Input: dimensioned drawing with shaded views. Units: mm. Origin: part minimum x, y, z. A direction names the side the tool comes from. Give positions to 0.01 mm unless a question says otherwise; leave off trailing zeros. Write each loop counter-clockwise with the first axis right and the second up, starting at its lowest first coordinate (ties: lowest second). Pieces come first, ordered by that corner, then holes. Notation, with made-up numbers: M 76.25,67.5 L 116.25,67.5 A22 cw 116.25,81.5 Z; hole C 8.25,8 d4. An arc over 180 degrees is marked long. Answer as a JSON object with one key per item and string values.
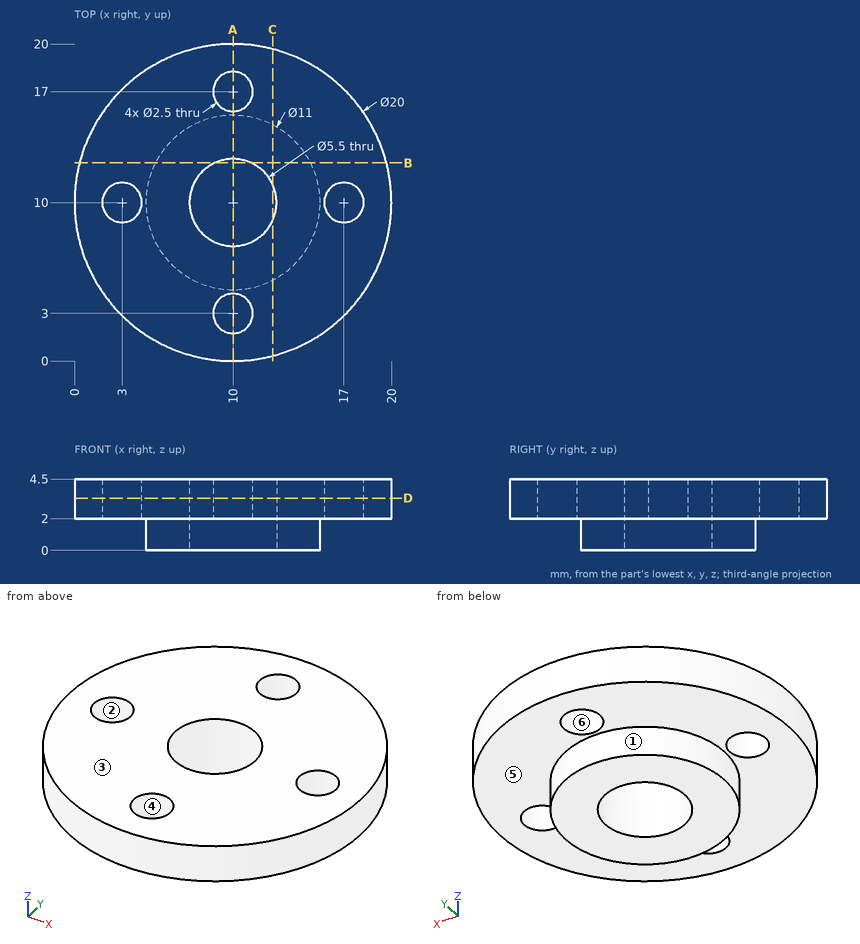
1) Pull-direction query (X, two-part tool) for the marked faces 1, 2, 3 and 4; classes: pulls with the +X half, pulls with the -X half, needs draft (parallel to the pull), parting line crosses it, or undercut.
Geometry check:
{"face 1": "parting line crosses it", "face 2": "undercut", "face 3": "needs draft", "face 4": "undercut"}
2) Set-up query: the marked faces 5 and 6. Return all of +Z, -Z, +X, -X, +Y, -Y with unobstructed straight access to the full face (end or side cutting, diameter ignored); none if empty.
Geometry check:
{"face 5": "-Z", "face 6": "+Z, -Z"}
3) Line query: line 1 (Y direction, x = 10, z = 3); line 2 (X direction, y = 9.75, z = 2.6); line 3 (Y direction, x = 17, z = 3.75). Output: solid intervals per line, ascending. Write a range as from..to.
Geometry check:
{"line 1": "y = 0..1.75, 4.25..7.25, 12.75..15.75, 18.25..20", "line 2": "x = 0..1.78, 4.22..7.26, 12.74..15.78, 18.22..20", "line 3": "y = 2.86..8.75, 11.25..17.14"}
4) Cut plane A-A on x = 10. Return loops of the section in (y, z).
Geometry check:
{"outline": "M 0,2 L 1.75,2 L 1.75,4.5 L 0,4.5 Z; M 4.25,2 L 4.5,2 L 4.5,0 L 7.25,0 L 7.25,4.5 L 4.25,4.5 Z; M 12.75,0 L 15.5,0 L 15.5,2 L 15.75,2 L 15.75,4.5 L 12.75,4.5 Z; M 18.25,2 L 20,2 L 20,4.5 L 18.25,4.5 Z"}
5) Contact query for a flat-ended pin moving along its axis: P1, Ø1.5, axis at y = 13.5, z = 4, coming from the +X side. Output: stop coordinate, or through.
Geometry check:
{"P1": "stops at x = 19.61"}
6) Cut plane B-B on y = 12.5. Return loops of the section in (x, z).
Geometry check:
{"outline": "M 0.32,2 L 5.1,2 L 5.1,0 L 8.85,0 L 8.85,4.5 L 0.32,4.5 Z; M 11.15,0 L 14.9,0 L 14.9,2 L 19.68,2 L 19.68,4.5 L 11.15,4.5 Z"}
7) Cut plane D-D on z = 3.3. Return loops of the section in (x, y).
Geometry check:
{"outline": "C 10,10 d20; hole C 3,10 d2.5; hole C 10,10 d5.5; hole C 10,3 d2.5; hole C 10,17 d2.5; hole C 17,10 d2.5"}
